Verification items for the finished model (mm, model axes). A direction names the side the tool comes from. Round coordinates to 2 decimals unless told otherwise and drop trailing zeros. Loops run counter-clockwise (first coordinate to the right, second up) from the corner with the lowest first, then second, coordinate; pieces in that order, holes last. Notation, with made-up numbers: (-21.5, 3.25) -> (-3.5, 3.25) arc R26 cw to (-3.5, 25.25) -> close; hole circle Ø1 at (-2.5, 87.25). An arc over 180 degrees is marked (long way). Write item = value, one per line.
```python
from build123d import *

# Parameters (mm, degrees)
SKETCH1_W           = 130
SKETCH1_H           = 83
SKETCH1_R           = 2
BOSS_EXTRUDE1_DEPTH = 2


with BuildPart() as part:
    # Sketch1 → Boss-Extrude1 (new body)
    with BuildSketch(Plane(origin=(0, 0, 0), x_dir=(1, 0, 0), z_dir=(0, 1, 0))):
        Rectangle(SKETCH1_W, SKETCH1_H)
        with Locations((13, 28.5)):
            Circle(SKETCH1_R, mode=Mode.SUBTRACT)
        with Locations((49.6, 28.5)):
            Circle(SKETCH1_R, mode=Mode.SUBTRACT)
        with Locations((49.6, -28.5)):
            Circle(SKETCH1_R, mode=Mode.SUBTRACT)
        with Locations((13, -28.5)):
            Circle(SKETCH1_R, mode=Mode.SUBTRACT)
        with Locations((-13, -28.5)):
            Circle(SKETCH1_R, mode=Mode.SUBTRACT)
        with Locations((-49.6, -28.5)):
            Circle(SKETCH1_R, mode=Mode.SUBTRACT)
        with Locations((-49.6, 28.5)):
            Circle(SKETCH1_R, mode=Mode.SUBTRACT)
        with Locations((-13, 28.5)):
            Circle(SKETCH1_R, mode=Mode.SUBTRACT)
        with Locations((-59, 35.5)):
            Circle(SKETCH1_R, mode=Mode.SUBTRACT)
        with Locations((59, 35.5)):
            Circle(SKETCH1_R, mode=Mode.SUBTRACT)
        with Locations((59, -35.5)):
            Circle(SKETCH1_R, mode=Mode.SUBTRACT)
        with Locations((-59, -35.5)):
            Circle(SKETCH1_R, mode=Mode.SUBTRACT)
        with BuildLine():
            Line((22.8, 25.5), (39.8, 25.5))
            ThreePointArc((39.8, 25.5), (48.8, 16.5), (39.8, 7.5))
            Line((39.8, 7.5), (22.8, 7.5))
            ThreePointArc((22.8, 7.5), (13.8, 16.5), (22.8, 25.5))
        make_face(mode=Mode.SUBTRACT)
        with BuildLine():
            Line((-22.8, 25.5), (-39.8, 25.5))
            ThreePointArc((-39.8, 25.5), (-48.8, 16.5), (-39.8, 7.5))
            Line((-39.8, 7.5), (-22.8, 7.5))
            ThreePointArc((-22.8, 7.5), (-13.8, 16.5), (-22.8, 25.5))
        make_face(mode=Mode.SUBTRACT)
    extrude(amount=BOSS_EXTRUDE1_DEPTH)


solid = part.part
```
(1) Draft check along Z on faces 1 (the face through (-1, 2, -1)), 2 (the face through (59.923, 0.986, -33.726)), 3 (the face through (-58.077, 0.986, -33.726)). Enter one of: released by +Z, released by -Z, zero draft, split by the parting line, or undercut.
Filled sheet:
face_1 = zero draft
face_2 = undercut
face_3 = undercut
(2) Sectioned sample at B-B, the plane z = 28.5. Record the cut outline in (x, y).
Filled sheet:
outline = (-65, 0) -> (-51.6, 0) -> (-51.6, 2) -> (-65, 2) -> close; (-47.6, 0) -> (-15, 0) -> (-15, 2) -> (-47.6, 2) -> close; (-11, 0) -> (11, 0) -> (11, 2) -> (-11, 2) -> close; (15, 0) -> (47.6, 0) -> (47.6, 2) -> (15, 2) -> close; (51.6, 0) -> (65, 0) -> (65, 2) -> (51.6, 2) -> close
(3) Set-up check for faces 4 (the face through (-1, 0, -1)), 5 (the face through (-13.802, 0.986, -16.302)): record each of +Z, -Z, +X, -X, +Y, -Y from which the full face is reachable in a straight line by a thin tool's end or side.
Filled sheet:
face_4 = +Z, -Z, +X, -X, -Y
face_5 = +Y, -Y
(4) Sectioned sample at A-A, the plane x = -33. Record the cut outline in (y, z), and give its area (3 significant figures).
Filled sheet:
outline = (0, -41.5) -> (2, -41.5) -> (2, -25.5) -> (0, -25.5) -> close; (0, -7.5) -> (2, -7.5) -> (2, 41.5) -> (0, 41.5) -> close
area = 130 mm2
(5) Material ranges on probe 1 along Z at (x, y) = (-49.6, 1.25); probe 2 along X at (y, z) = (0.2, -16.5); probe 3 along X at (y, z) = (1.35, 28.5), recorded low to high. Write a range as from..to.
Filled sheet:
probe_1 = -41.5..-30.5, -26.5..26.5, 30.5..41.5
probe_2 = -65..-48.8, -13.8..13.8, 48.8..65
probe_3 = -65..-51.6, -47.6..-15, -11..11, 15..47.6, 51.6..65
(6) Sectioned sample at C-C, the plane z = -16.5. Record the cut outline in (x, y), and give its area (3 significant figures).
Filled sheet:
outline = (-65, 0) -> (-48.8, 0) -> (-48.8, 2) -> (-65, 2) -> close; (-13.8, 0) -> (13.8, 0) -> (13.8, 2) -> (-13.8, 2) -> close; (48.8, 0) -> (65, 0) -> (65, 2) -> (48.8, 2) -> close
area = 120 mm2
(7) Sectioned sample at D-D, the plane y = 1.6. Count the separate pieces of the cut face and the enclosed holes in it, and give its area (3 significant figures).
Filled sheet:
separate_pieces = 1
enclosed_holes = 14
area = 9,520 mm2
